Input: part model. Units: mm. Frame: model coordinates. A direction names the side the tool comes from. Round coordinates to 2 decimals unless told otherwise and drop trailing zeros. Loops run counter-clockwise (first coordinate to the right, second up) from the corner with the lowest first, then second, coordinate; pieces in that order, holes last.
(1) Access query for faces 4 (the face through (0, 1, 0)), 5 (the face through (-12.385, 29.14, 5.751)), 6 (the face through (-7.615, -29.14, 5.751)). Directions: +Z, -Z, +X, -X, +Y, -Y. A direction counts if a zero-diameter tool reaches every point of the face in a straight line with its end or side. Return the directions, or none.
(2) Draft query along Y for faces 1 (the face through (-10.54, 16.56, 4.93)), 2 (the face through (0, -39, 5)), 3 (the face through (12.385, -29.14, 5.751)). Return one class per face: released by +Y, released by -Y, zero draft, split by the parting line, or undercut.
(3) First-contact query: pin 1 Ø1.5 at (x, z) = (8.5, 4) entering from -Y. Flat tip, straight axial feed; report the tip coordinate or a pass-through.
(4) Cut plane A-A, the plane x = -10. Output: boundary loops of the cut face in (y, z), and give its area (3 significant figures).
(5) Cut plane C-C, the plane y = 18. Output: boundary loops of the cut face in (x, z), and give its area (3 significant figures).
(6) Cut plane D-D, the plane y = 34. Output: boundary loops of the cut face in (x, z), and give its area (3 significant figures).
(7) Cut plane B-B, the plane z = 5. Output: boundary loops of the cut face in (x, y), and give its area (3 significant figures).
(8) Line query: line 1 (X direction, y = -25.75, z = 5); line 2 (Z direction, x = 10, y = -32.25); line 3 (X direction, y = 31.5, z = 3.25). Output: solid intervals per line, ascending.
from build123d import *

# Parameters (mm, degrees)
F0_W     = 30
F0_H     = 78
F0_R     = 2.5
F1_DEPTH = 10
F2_R     = 2.5
F3_DEPTH = 20
F4_R     = 2.5
F5_DEPTH = 20


with BuildPart() as f1:
    # F0 (on Top) → F1 (new body)
    with BuildSketch(Plane.XY):
        Rectangle(F0_W, F0_H)
        with Locations((-10, -19)):
            Circle(F0_R, mode=Mode.SUBTRACT)
        with Locations((10, -19)):
            Circle(F0_R, mode=Mode.SUBTRACT)
        with Locations((-10, 19)):
            Circle(F0_R, mode=Mode.SUBTRACT)
        with Locations((10, 19)):
            Circle(F0_R, mode=Mode.SUBTRACT)
    extrude(amount=F1_DEPTH)

    # F2 (on face) → F3 (cut)
    with BuildSketch(Plane(origin=(0, 39, 0), x_dir=(-1, 0, 0), z_dir=(0, 1, 0))):
        with Locations((-10, 5)):
            Circle(F2_R)
        with Locations((10, 5)):
            Circle(F2_R)
    extrude(amount=-F3_DEPTH, mode=Mode.SUBTRACT)

    # F4 (on face) → F5 (cut)
    with BuildSketch(Plane.XZ.offset(39)):
        with Locations((-10, 5)):
            Circle(F4_R)
        with Locations((10, 5)):
            Circle(F4_R)
    extrude(amount=-F5_DEPTH, mode=Mode.SUBTRACT)


solid = f1.part
Reported:
1. face 4: -Z, +X, -X, +Y, -Y
1. face 5: +Y
1. face 6: -Y
2. face 1: undercut
2. face 2: released by -Y
2. face 3: zero draft
3. pin 1: stops at y = -39
4. outline: (-39, 0) - (-21.5, 0) - (-21.5, 2.5) - (-39, 2.5) - close; (-39, 7.5) - (-21.5, 7.5) - (-21.5, 10) - (-39, 10) - close; (-16.5, 0) - (16.5, 0) - (16.5, 10) - (-16.5, 10) - close; (21.5, 0) - (39, 0) - (39, 2.5) - (21.5, 2.5) - close; (21.5, 7.5) - (39, 7.5) - (39, 10) - (21.5, 10) - close
4. area: 505 mm2
5. outline: (-15, 0) - (-12.29, 0) - (-12.29, 10) - (-15, 10) - close; (-7.71, 0) - (7.71, 0) - (7.71, 10) - (-7.71, 10) - close; (12.29, 0) - (15, 0) - (15, 10) - (12.29, 10) - close
5. area: 208 mm2
6. outline: (-15, 0) - (15, 0) - (15, 10) - (-15, 10) - close; hole circle Ø5 at (-10, 5); hole circle Ø5 at (10, 5)
6. area: 261 mm2
7. outline: (-15, -39) - (-12.5, -39) - (-12.5, -19) arc R2.5 cw to (-7.5, -19) - (-7.5, -39) - (7.5, -39) - (7.5, -19) arc R2.5 cw to (12.5, -19) - (12.5, -39) - (15, -39) - (15, 39) - (12.5, 39) - (12.5, 19) arc R2.5 cw to (7.5, 19) - (7.5, 39) - (-7.5, 39) - (-7.5, 19) arc R2.5 cw to (-12.5, 19) - (-12.5, 39) - (-15, 39) - close
7. area: 1,900 mm2
8. line 1: x = -15 to -12.5, -7.5 to 7.5, 12.5 to 15
8. line 2: z = 0 to 2.5, 7.5 to 10
8. line 3: x = -15 to -11.79, -8.21 to 8.21, 11.79 to 15
